Design review of the part shown in the three views and the two pictorial views. Dimensions are in mm from the part's minimum x, y and z. A direction names the side the tool comes from. Coordinates: 2 decimals unless noted, no trailing zeros. Loops run counter-clockwise (first coordinate to the right, second up) from the corner with the lowest first, then second, coordinate; pieces in that order, holes last. Notation, with made-up numbers: (37, -7) -> (63, -7) arc R17 cw to (63, 17) -> close; hole circle Ø8 at (43.25, 68). An arc over 180 degrees is marked (long way). Answer in a Markdown table with one row per item.
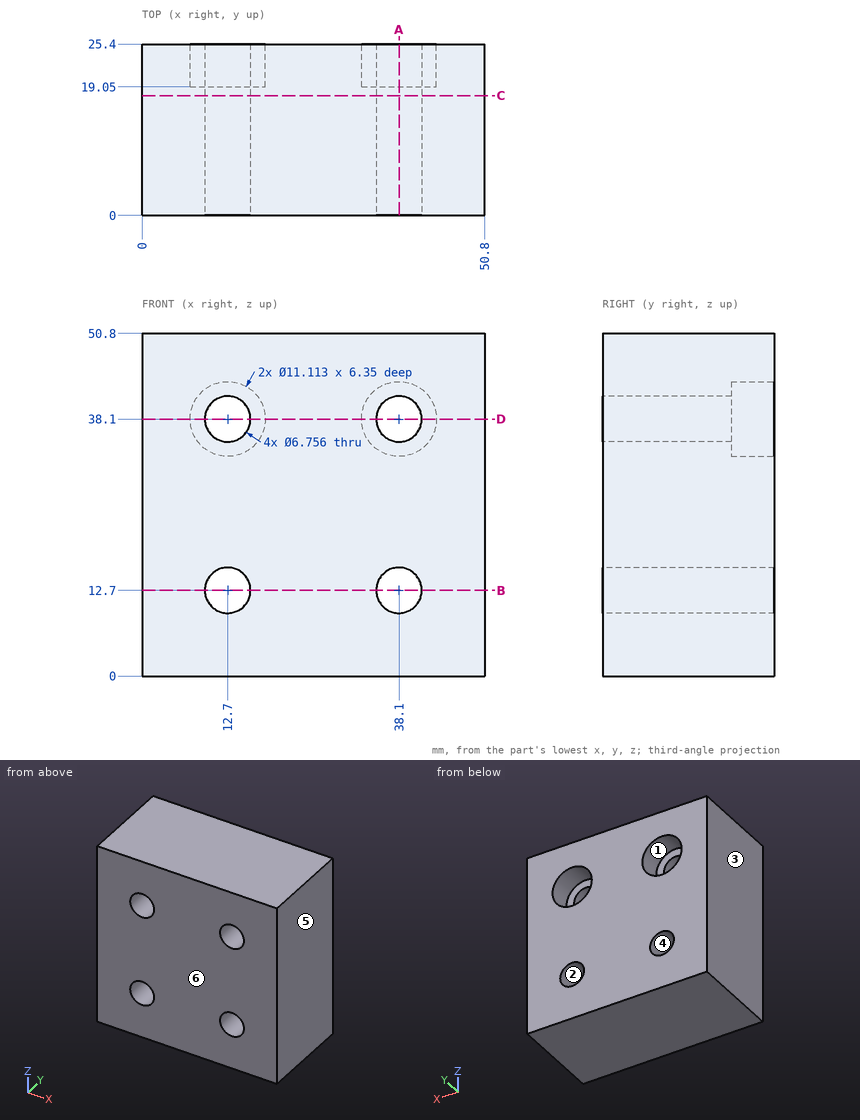
Item 1: Insertion check: pin 1 (9 mm diameter, centred on x = 38.1, z = 38.1, fed in from +Y); pin 2 (4 mm diameter, centred on x = 12.7, z = 38.1, fed in from +Y). Each pin has a flat end and moves straight along its axis. Give the tip position at first contact, or say it passes through.
Worked answers:
| item | result |
|---|---|
| pin 1 | y = 19.05 |
| pin 2 | through |
Item 2: Take a section at A-A, the plane x = 38.1. State the section outline as (y, z) points.
Worked answers:
| item | result |
|---|---|
| outline | (0, 0) -> (25.4, 0) -> (25.4, 9.32) -> (0, 9.32) -> close; (0, 16.08) -> (25.4, 16.08) -> (25.4, 32.54) -> (19.05, 32.54) -> (19.05, 34.72) -> (0, 34.72) -> close; (0, 41.48) -> (19.05, 41.48) -> (19.05, 43.66) -> (25.4, 43.66) -> (25.4, 50.8) -> (0, 50.8) -> close |
Item 3: For L1, parallel to Z at x = 38.1, y = 13; L2, parallel to Z at x = 38.1, y = 23.25; L3, parallel to X at y = 4.25, z = 14.5, list the stretches that pass through material, from the lowest coordinate up.
Worked answers:
| item | result |
|---|---|
| L1 | 0 to 9.32, 16.08 to 34.72, 41.48 to 50.8 |
| L2 | 0 to 9.32, 16.08 to 32.54, 43.66 to 50.8 |
| L3 | 0 to 9.84, 15.56 to 35.24, 40.96 to 50.8 |
Item 4: Take a section at C-C, the plane y = 17.75. State the section outline as (x, z) points.
Worked answers:
| item | result |
|---|---|
| outline | (0, 0) -> (50.8, 0) -> (50.8, 50.8) -> (0, 50.8) -> close; hole circle Ø6.76 at (12.7, 12.7); hole circle Ø6.76 at (12.7, 38.1); hole circle Ø6.76 at (38.1, 12.7); hole circle Ø6.76 at (38.1, 38.1) |
Item 5: Take a section at B-B, the plane z = 12.7. State the section outline as (x, y) points, and give its area (3 significant figures).
Worked answers:
| item | result |
|---|---|
| outline | (0, 0) -> (9.32, 0) -> (9.32, 25.4) -> (0, 25.4) -> close; (16.08, 0) -> (34.72, 0) -> (34.72, 25.4) -> (16.08, 25.4) -> close; (41.48, 0) -> (50.8, 0) -> (50.8, 25.4) -> (41.48, 25.4) -> close |
| area | 947 mm² |
Item 6: For the marked faces 1 and 2, list the 3-axis set-ups (+Z, -Z, +X, -X, +Y, -Y) from which the entire face can be reached by the end or side of a thin tool; tool diameter is ignored.
Worked answers:
| item | result |
|---|---|
| face 1 | +Y |
| face 2 | +Y, -Y |
Item 7: Take a section at D-D, the plane z = 38.1. State the section outline as (x, y) points.
Worked answers:
| item | result |
|---|---|
| outline | (0, 0) -> (9.32, 0) -> (9.32, 19.05) -> (7.14, 19.05) -> (7.14, 25.4) -> (0, 25.4) -> close; (16.08, 0) -> (34.72, 0) -> (34.72, 19.05) -> (32.54, 19.05) -> (32.54, 25.4) -> (18.26, 25.4) -> (18.26, 19.05) -> (16.08, 19.05) -> close; (41.48, 0) -> (50.8, 0) -> (50.8, 25.4) -> (43.66, 25.4) -> (43.66, 19.05) -> (41.48, 19.05) -> close |
Item 8: The part is to be moulded in two halves that separate along X. For the marked faces 3, 4, 5 and 6, say which applies: +X half, -X half, draft (parallel to the pull), parting line (faces both ways), or undercut.
Worked answers:
| item | result |
|---|---|
| face 3 | -X half |
| face 4 | undercut |
| face 5 | +X half |
| face 6 | draft |
